Input: dimensioned drawing with shaded views. Units: mm. Origin: part minimum x, y, z. Round coordinates to 2 decimals unless told otherwise and drop trailing zeros. Loops run counter-clockwise (first coordinate to the right, second up) from the corner with the lowest first, then second, coordinate; pieces in that order, holes last. Notation, with made-up numbers: (29.5, 87.5) -> (85.5, 87.5) arc R20 cw to (85.5, 122.5) -> close; hole circle Ø9 at (69, 31). An arc over 180 degrees is marked (long way). Answer as a JSON object with one key per item and string values.
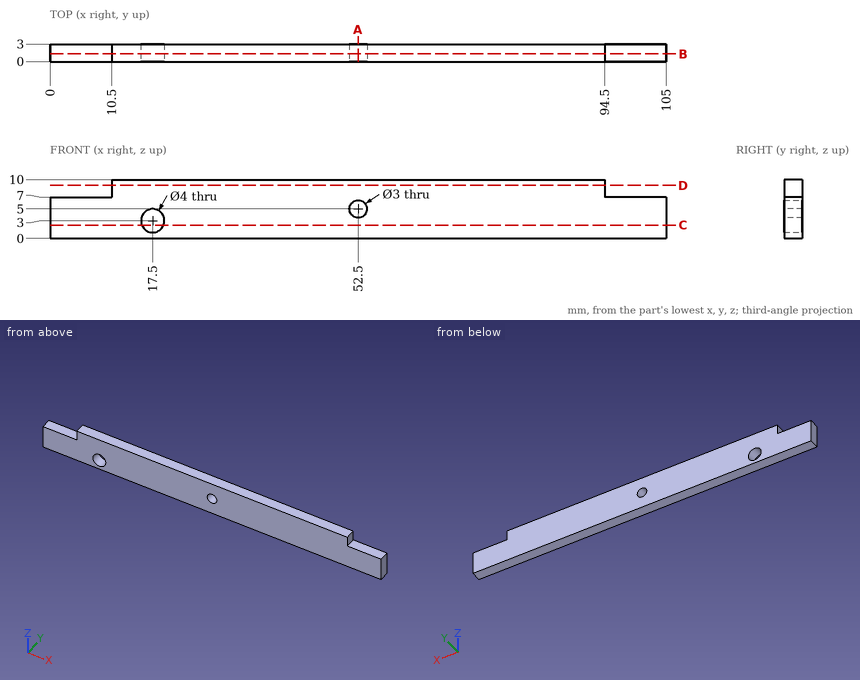
1) Section C-C, the plane z = 2.25. Output: boundary loops of the cut face in (x, y).
Output:
{"outline": "(0, 0) -> (15.65, 0) -> (15.65, 3) -> (0, 3) -> close; (19.35, 0) -> (105, 0) -> (105, 3) -> (19.35, 3) -> close"}
2) Section D-D, the plane z = 9. Output: boundary loops of the cut face in (x, y).
Output:
{"outline": "(10.5, 0) -> (94.5, 0) -> (94.5, 3) -> (10.5, 3) -> close"}
3) Contact query for flat-ended pins moving along their axis: P1, Ø2.5, axis at x = 52.5, z = 5, coming from the -Y side; P2, Ø1.5, axis at y = 1, z = 8.5, coming from the +X side; P3, Ø1.5, axis at x = 6, y = 1, coming from the +Z side. Output: stop coordinate, or through.
Output:
{"P1": "passes through", "P2": "stops at x = 94.5", "P3": "stops at z = 7"}
4) Section B-B, the plane y = 1.3. Output: boundary loops of the cut face in (x, z).
Output:
{"outline": "(0, 0) -> (105, 0) -> (105, 7) -> (94.5, 7) -> (94.5, 10) -> (10.5, 10) -> (10.5, 7) -> (0, 7) -> close; hole circle Ø4 at (17.5, 3); hole circle Ø3 at (52.5, 5)"}
5) Ray query, probe 1 along X at (y, z) = (1.1, 3); probe 2 along X at (y, z) = (1.75, 9.5); probe 3 along X at (y, z) = (0.35, 4.25). Return the intervals inside material, ascending.
Output:
{"probe 1": "x = 0 to 15.5, 19.5 to 105", "probe 2": "x = 10.5 to 94.5", "probe 3": "x = 0 to 15.94, 19.06 to 51.2, 53.8 to 105"}
6) Section A-A, the plane x = 52.5. Output: boundary loops of the cut face in (y, z).
Output:
{"outline": "(0, 0) -> (3, 0) -> (3, 3.5) -> (0, 3.5) -> close; (0, 6.5) -> (3, 6.5) -> (3, 10) -> (0, 10) -> close"}
